```python
from build123d import *

# Parameters (mm, degrees)
SKETCH_1_R               = 2.5
SKETCH_1_R_2             = 1.5
SKETCH_1_W               = 10
SKETCH_1_H               = 6
EXTRUDE_1_DEPTH          = 6
FILLET_1_R               = 3.5
FILLET_2_R               = 3
CUT_EXTRUDE_1_DEPTH      = 403.661147865
CUT_EXTRUDE_1_DEPTH_BACK = 403.661147865
SKETCH_2_R               = 1.5


with BuildPart() as part:
    # Эскиз1 → Бобышка-Вытянуть1 (new body)
    with BuildSketch(Plane.XY):
        with BuildLine():
            Line((94, -65.75), (94, -22.45))
            Line((94, -22.45), (83, -22.45))
            Line((83, -22.45), (83, -23.925))
            Line((83, -23.925), (79.2, -23.925))
            Line((79.2, -23.925), (79.2, -22.45))
            Line((79.2, -22.45), (75, -22.45))
            Line((75, -22.45), (75, -17.55))
            Line((75, -17.55), (79.2, -17.55))
            Line((79.2, -17.55), (79.2, -16.075))
            Line((79.2, -16.075), (83, -16.075))
            Line((83, -16.075), (83, -17.55))
            Line((83, -17.55), (94, -17.55))
            Line((94, -17.55), (94, 9))
            Line((94, 9), (59.275, 9))
            Line((59.275, 9), (59.275, -61))
            Line((59.275, -61), (29.275, -61))
            Line((29.275, -61), (29.275, 9))
            Line((29.275, 9), (19.232050808, 9))
            Line((19.232050808, 9), (17.5, 12))
            Line((17.5, 12), (-17.5, 12))
            Line((-17.5, 12), (-19.232050808, 9))
            Line((-19.232050808, 9), (-29.275, 9))
            Line((-29.275, 9), (-29.275, -61))
            Line((-29.275, -61), (-59.275, -61))
            Line((-59.275, -61), (-59.275, 9))
            Line((-59.275, 9), (-100, 9))
            Line((-100, 9), (-100, -390))
            Line((-100, -390), (19, -390))
            Line((19, -390), (19, -351))
            ThreePointArc((19, -351), (31.594408409, -320.594408409), (62, -308))
            Line((62, -308), (94, -308))
            Line((94, -308), (94, -275.45))
            Line((94, -275.45), (83, -275.45))
            Line((83, -275.45), (83, -276.925))
            Line((83, -276.925), (79.2, -276.925))
            Line((79.2, -276.925), (79.2, -275.45))
            Line((79.2, -275.45), (75, -275.45))
            Line((75, -275.45), (75, -270.55))
            Line((75, -270.55), (79.2, -270.55))
            Line((79.2, -270.55), (79.2, -269.075))
            Line((79.2, -269.075), (83, -269.075))
            Line((83, -269.075), (83, -270.55))
            Line((83, -270.55), (94, -270.55))
            Line((94, -270.55), (94, -227.25))
            Line((94, -227.25), (100, -227.25))
            Line((100, -227.25), (100, -192.25))
            Line((100, -192.25), (94, -192.25))
            Line((94, -192.25), (94, -148.95))
            Line((94, -148.95), (83, -148.95))
            Line((83, -148.95), (83, -150.425))
            Line((83, -150.425), (79.2, -150.425))
            Line((79.2, -150.425), (79.2, -148.95))
            Line((79.2, -148.95), (75, -148.95))
            Line((75, -148.95), (75, -144.05))
            Line((75, -144.05), (79.2, -144.05))
            Line((79.2, -144.05), (79.2, -142.575))
            Line((79.2, -142.575), (83, -142.575))
            Line((83, -142.575), (83, -144.05))
            Line((83, -144.05), (94, -144.05))
            Line((94, -144.05), (94, -100.75))
            Line((94, -100.75), (100, -100.75))
            Line((100, -100.75), (100, -65.75))
            Line((100, -65.75), (94, -65.75))
        make_face()
        with Locations((-70.1375, 3)):
            Circle(SKETCH_1_R, mode=Mode.SUBTRACT)
        with Locations((0, 3)):
            Circle(SKETCH_1_R, mode=Mode.SUBTRACT)
        with Locations(Location((70.1375, 3, 0), (0, 0, 180))):
            Circle(SKETCH_1_R, mode=Mode.SUBTRACT)
        with Locations((-70.1375, -382)):
            Circle(SKETCH_1_R, mode=Mode.SUBTRACT)
        with Locations((0, -382)):
            Circle(SKETCH_1_R, mode=Mode.SUBTRACT)
        with Locations((-70.1375, -323)):
            Circle(SKETCH_1_R, mode=Mode.SUBTRACT)
        with Locations((0, -323)):
            Circle(SKETCH_1_R, mode=Mode.SUBTRACT)
        with Locations((-44.275, -67)):
            Circle(SKETCH_1_R_2, mode=Mode.SUBTRACT)
        with Locations((-65.275, -7)):
            Circle(SKETCH_1_R_2, mode=Mode.SUBTRACT)
        with Locations(Location((-23.275, -7, 0), (0, 0, 180))):
            Circle(SKETCH_1_R_2, mode=Mode.SUBTRACT)
        with Locations(Location((44.275, -67, 0), (0, 0, 180))):
            Circle(SKETCH_1_R_2, mode=Mode.SUBTRACT)
        with Locations((23.275, -7)):
            Circle(SKETCH_1_R_2, mode=Mode.SUBTRACT)
        with Locations(Location((65.275, -7, 0), (0, 0, 180))):
            Circle(SKETCH_1_R_2, mode=Mode.SUBTRACT)
        with Locations((15.8625, 3)):
            Rectangle(SKETCH_1_W, SKETCH_1_H, mode=Mode.SUBTRACT)
        with Locations((-15.8625, 3)):
            Rectangle(SKETCH_1_W, SKETCH_1_H, mode=Mode.SUBTRACT)
        with Locations((-86, 3)):
            Rectangle(SKETCH_1_W, SKETCH_1_H, mode=Mode.SUBTRACT)
        with Locations((86, 3)):
            Rectangle(SKETCH_1_W, SKETCH_1_H, mode=Mode.SUBTRACT)
        with Locations((-86, -382)):
            Rectangle(SKETCH_1_W, SKETCH_1_H, mode=Mode.SUBTRACT)
        with Locations((-15.8625, -382)):
            Rectangle(SKETCH_1_W, SKETCH_1_H, mode=Mode.SUBTRACT)
        with Locations((-86, -323)):
            Rectangle(SKETCH_1_W, SKETCH_1_H, mode=Mode.SUBTRACT)
        with Locations((-15.8625, -323)):
            Rectangle(SKETCH_1_W, SKETCH_1_H, mode=Mode.SUBTRACT)
    extrude(amount=EXTRUDE_1_DEPTH)

    # Скругление1
    fillet_1_edges = [part.edges().sort_by_distance(p)[0] for p in [
        (19, -390, 3),
        (-100, -390, 3),
    ]]
    fillet(fillet_1_edges, radius=FILLET_1_R)

    # Скругление2
    fillet_2_edges = [part.edges().sort_by_distance(p)[0] for p in [
        (94, -308, 3),
        (-100, 9, 3),
        (-59.275, -61, 3),
        (-29.275, -61, 3),
        (29.275, -61, 3),
        (59.275, -61, 3),
    ]]
    fillet(fillet_2_edges, radius=FILLET_2_R)

    # Эскиз2 → Вырез-Вытянуть1 (cut, two sides: drawn at the far end of the back side and taken through both)
    with BuildSketch(Plane.XY.offset(6).offset(-CUT_EXTRUDE_1_DEPTH_BACK)):
        with Locations((15, -351)):
            Circle(SKETCH_2_R)
        with Locations((28.765981284, -317.765981284)):
            Circle(SKETCH_2_R)
        with Locations((62, -304)):
            Circle(SKETCH_2_R)
    extrude(amount=CUT_EXTRUDE_1_DEPTH + CUT_EXTRUDE_1_DEPTH_BACK, mode=Mode.SUBTRACT)


solid = part.part
```
Geometry check sheet. Reference: the model listing, model coordinates, mm. Round coordinates to 2 decimals unless told otherwise and drop trailing zeros. Order: outer loops, then holes, each group sorted by start corner. A loop starts at its lowest first (then second) coordinate and runs counter-clockwise, first axis right, second up. Notation, with made-up numbers: (-17, 37.5) - (18, 37.5) arc R20 cw to (18, 65.5) - close; hole circle Ø5 at (35, 76). An arc over 180 degrees is marked (long way). Use a Markdown table: item, result. Add a question column.
1) Section check B-B (z = 3). Count the separate pieces of the cut face and the enclosed holes in it, then the cut area to 3 significant figures.
2) Thickness scan on line 1 along X through (y, z) = (-382, 3.05); line 2 along Y through (x, z) = (-70.5, 4.8); line 3 along X through (y, z) = (-67, 1.25) (3 decimals). Record the ranges inside material, lowest first.
3) Section check A-A (y = -134). Record the cut outline in (x, z).
4) Gauge pin test, flat ends, axial feed: P1, Ø2, axis at x = -26.5, z = 5, coming from the +Y side; P2, Ø3, axis at y = -31, z = 3, coming from the +X side; P3, Ø2.5, axis at x = 44.275, y = -67, coming from the -Z side; P4, Ø2.5, axis at y = -272, z = 3.5, coming from the +X side. Record the tip position at first contact, or that the pin passes through.
Established:
| question | item | result |
|---|---|---|
| 1 | separate pieces | 1 |
| 1 | enclosed holes | 24 |
| 1 | area | 67,000 mm2 |
| 2 | line 1 | -100 to -91, -81 to -72.64, -67.64 to -20.86, -10.86 to -2.5, 2.5 to 19 |
| 2 | line 2 | -390 to -384.47, -379.53 to -325.47, -320.53 to 0.53, 5.47 to 9 |
| 2 | line 3 | -100 to -45.775, -42.775 to 42.775, 45.775 to 100 |
| 3 | outline | (-100, 0) - (94, 0) - (94, 6) - (-100, 6) - close |
| 4 | P1 | y = 9 |
| 4 | P2 | x = 94 |
| 4 | P3 | through |
| 4 | P4 | x = 75 |
